Verification items for the finished model (mm, model axes). A direction names the side the tool comes from. Give positions to 0.01 mm unless a question says otherwise; leave off trailing zeros. Loops run counter-clockwise (first coordinate to the right, second up) from the corner with the lowest first, then second, coordinate; pieces in that order, holes last. Notation, with made-up numbers: (-18, 83.25) -> (20, 83.25) arc R3 ccw to (20, 88.25) -> close; hole circle Ø10 at (30, 88). An arc over 180 degrees is marked (long way). Answer in a Markdown table with one row per item. Add a question column.
Q1. Material ranges on probe 1 along X at (y, z) = (-3.25, 0.4); probe 2 along Y at (x, z) = (-5, 0.6); probe 3 along Y at (x, z) = (1.25, -0.5), recorded low to high.
Q2. Section check A-A on y = 0. Enter the section's corners in (x, z) (3 decimals).
Q3. Section check D-D on x = -8.5. Enter the section's corners in (y, z), and give its area (3 significant figures).
Q4. Section check B-B on z = -0.1. Enter the section's corners in (x, y) (3 decimals).
Q5. Release check for a two-part mould opening along X. For faces 3 (the face through (-7.559, -5.796, 0.011)), 4 (the face through (-2.3, -6.2, -0.8)), 5 (the face through (3.219, -5.474, -0.011)) record: pulls with the +X half, pulls with the -X half, needs draft (parallel to the pull), parting line crosses it, or undercut.
Q6. Set-up check for faces 1 (the face through (-2.3, -6.2, 0.8)), 2 (the face through (-3.131, -5.525, -0.011)): record each of +Z, -Z, +X, -X, +Y, -Y from which the full face is reachable in a straight line by a thin tool's end or side.
Q7. Section check C-C on x = 1. Enter the section's corners in (y, z).
Q8. Gauge pin test, flat end, axial feed: P1, Ø3, axis at x = -3.5, y = 3, coming from the -Z side. Record the tip position at first contact, or that the pin passes through.
Autodesk Inventor part; units mm, degrees
ref_plane "YZ Plane" through (0, 0, 0) normal (1, 0, 0) x (0, 1, 0)
ref_plane "XZ Plane" through (0, 0, 0) normal (0, 1, 0) x (-1, 0, 0)
ref_plane "XY Plane" through (0, 0, 0) normal (0, 0, 1) x (1, 0, 0)
sketch "Sketch1" plane through (0, 0, 0) normal (0, 0, 1) x (1, 0, 0)
  circle A0 centre (0, 0) radius 9.525
  line L0 (0, 7.3323) -> (6.35, 3.6662)
  line L1 (6.35, 3.6662) -> (6.35, -3.6662)
  line L2 (6.35, -3.6662) -> (0, -7.3323)
  line L3 (0, -7.3323) -> (-6.35, -3.6662)
  line L4 (-6.35, -3.6662) -> (-6.35, 3.6662)
  line L5 (-6.35, 3.6662) -> (0, 7.3323)
  dimension "d0" = 19.05
  dimension "d2" = 12.7
extrude "Extrusion1" add sketch "Sketch1" along normal mid plane 1.6002
properties part number "500 Hex Spacer x250" material "Nylon 6/6"
Taken from the geometry:
| question | item | result |
|---|---|---|
| 1 | probe 1 | x = -8.95 to -6.35, 6.35 to 8.95 |
| 1 | probe 2 | y = -8.11 to -4.45, 4.45 to 8.11 |
| 1 | probe 3 | y = -9.44 to -6.61, 6.61 to 9.44 |
| 2 | outline | (-9.525, -0.8) -> (-6.35, -0.8) -> (-6.35, 0.8) -> (-9.525, 0.8) -> close; (6.35, -0.8) -> (9.525, -0.8) -> (9.525, 0.8) -> (6.35, 0.8) -> close |
| 3 | outline | (-4.3, -0.8) -> (4.3, -0.8) -> (4.3, 0.8) -> (-4.3, 0.8) -> close |
| 3 | area | 13.8 mm² |
| 4 | outline | circle Ø19.05 at (0, 0); hole (-6.35, -3.666) -> (0, -7.332) -> (6.35, -3.666) -> (6.35, 3.666) -> (0, 7.332) -> (-6.35, 3.666) -> close |
| 5 | face 3 | parting line crosses it |
| 5 | face 4 | needs draft |
| 5 | face 5 | undercut |
| 6 | face 1 | +Z, +X, -X, +Y, -Y |
| 6 | face 2 | +Z, -Z |
| 7 | outline | (-9.47, -0.8) -> (-6.75, -0.8) -> (-6.75, 0.8) -> (-9.47, 0.8) -> close; (6.75, -0.8) -> (9.47, -0.8) -> (9.47, 0.8) -> (6.75, 0.8) -> close |
| 8 | P1 | passes through |
